Verification items for this drawing (mm, ordinates from the low corner). A direction names the side the tool comes from. Coordinates: 2 decimals unless noted, no trailing zeros. Loops run counter-clockwise (first coordinate to the right, second up) from the corner with the lowest first, then second, coordinate; pieces in that order, holes last. Notation, with made-up numbers: M 63.25,56 L 86.25,56 A25 ccw 86.25,81 Z; hole C 34.25,-20.5 d3. An arc over 180 degrees is marked long. Return JSON: item names as keys, results as strings.
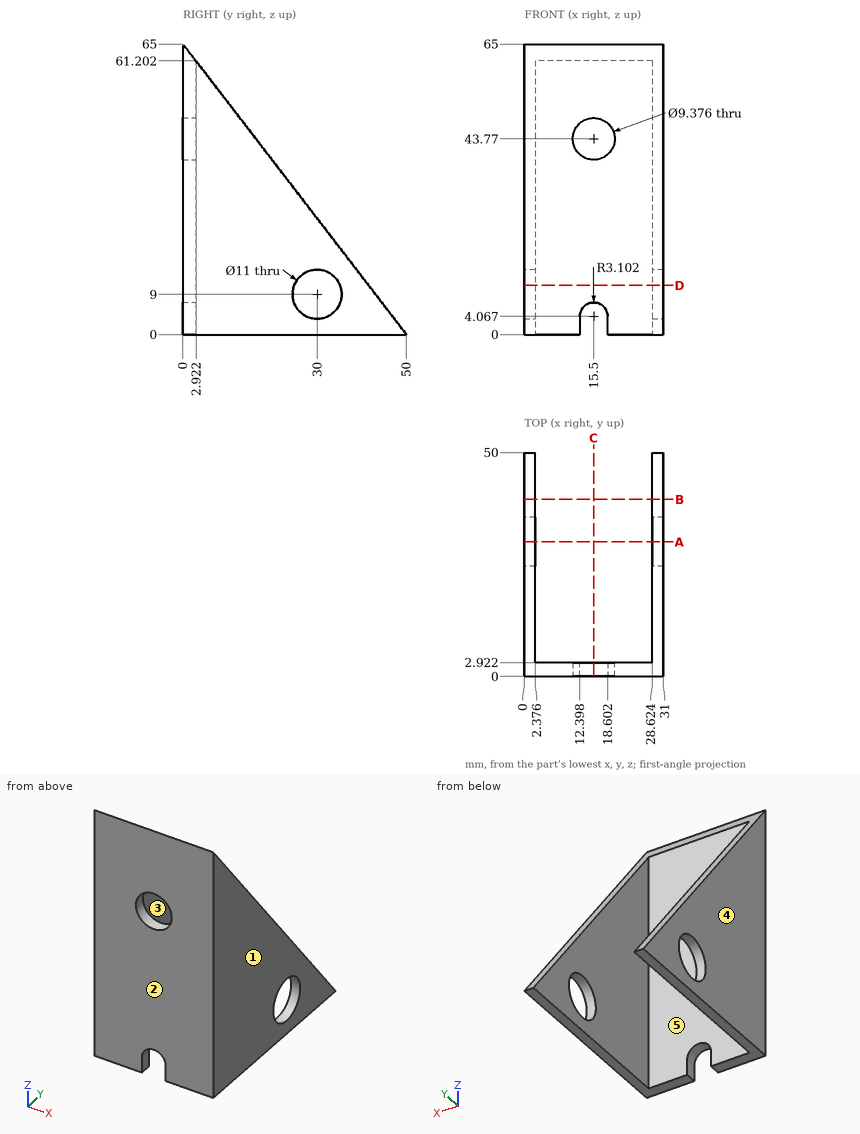
1) Go/stop test with flat-tipped pins: pin 1 Ø9 at (y, z) = (30, 9) entering from +X; pin 2 Ø13 at (x, z) = (9.5, 38) entering from +Y. Record where each tip stops, or that it passes through.
Answers:
{"pin 1": "through", "pin 2": "y = 2.92"}
2) Section check A-A on y = 30. Record the cut outline in (x, z).
Answers:
{"outline": "M 0,0 L 2.38,0 L 2.38,3.5 L 0,3.5 Z; M 0,14.5 L 2.38,14.5 L 2.38,26 L 0,26 Z; M 28.62,0 L 31,0 L 31,3.5 L 28.62,3.5 Z; M 28.62,14.5 L 31,14.5 L 31,26 L 28.62,26 Z"}
3) Scan lines: line 1 along X through (y, z) = (34, 20.5); line 2 along Y through (x, z) = (30.1, 9) (1 decimal); line 3 along Y through (x, z) = (24, 29.5). Record each from-to range of solid material in increasing order. Write a range as [from, to].
Answers:
{"line 1": "[0, 2.38], [28.62, 31]", "line 2": "[0, 24.5], [35.5, 43.1]", "line 3": "[0, 2.92]"}
4) Draft check along X on the marked faces 1, 2 and 3. Enter one of: +X half, -X half, draft (parallel to the pull), parting line (faces both ways), or undercut.
Answers:
{"face 1": "+X half", "face 2": "draft", "face 3": "undercut"}
5) Section check D-D on z = 11. Record the cut outline in (x, y).
Answers:
{"outline": "M 0,0 L 31,0 L 31,24.88 L 28.62,24.88 L 28.62,2.92 L 2.38,2.92 L 2.38,24.88 L 0,24.88 Z; M 0,35.12 L 2.38,35.12 L 2.38,41.54 L 0,41.54 Z; M 28.62,35.12 L 31,35.12 L 31,41.54 L 28.62,41.54 Z"}
6) Section check C-C on x = 15.5. Record the cut outline in (y, z), then the cut area to 3 significant figures.
Answers:
{"outline": "M 0,7.17 L 2.92,7.17 L 2.92,39.08 L 0,39.08 Z; M 0,48.46 L 2.92,48.46 L 2.92,61.2 L 0,65 Z", "area": "136 mm²"}
7) Section check B-B on y = 39.5. Record the cut outline in (x, z).
Answers:
{"outline": "M 0,0 L 2.38,0 L 2.38,13.65 L 0,13.65 Z; M 28.62,0 L 31,0 L 31,13.65 L 28.62,13.65 Z"}
8) Set-up check for the marked faces 4 and 5: record each of +Z, -Z, +X, -X, +Y, -Y from which the full face is reachable in a straight line by a thin tool's end or side.
Answers:
{"face 4": "+Z, -Z, -X, +Y, -Y", "face 5": "+Z, -Z, +Y"}
